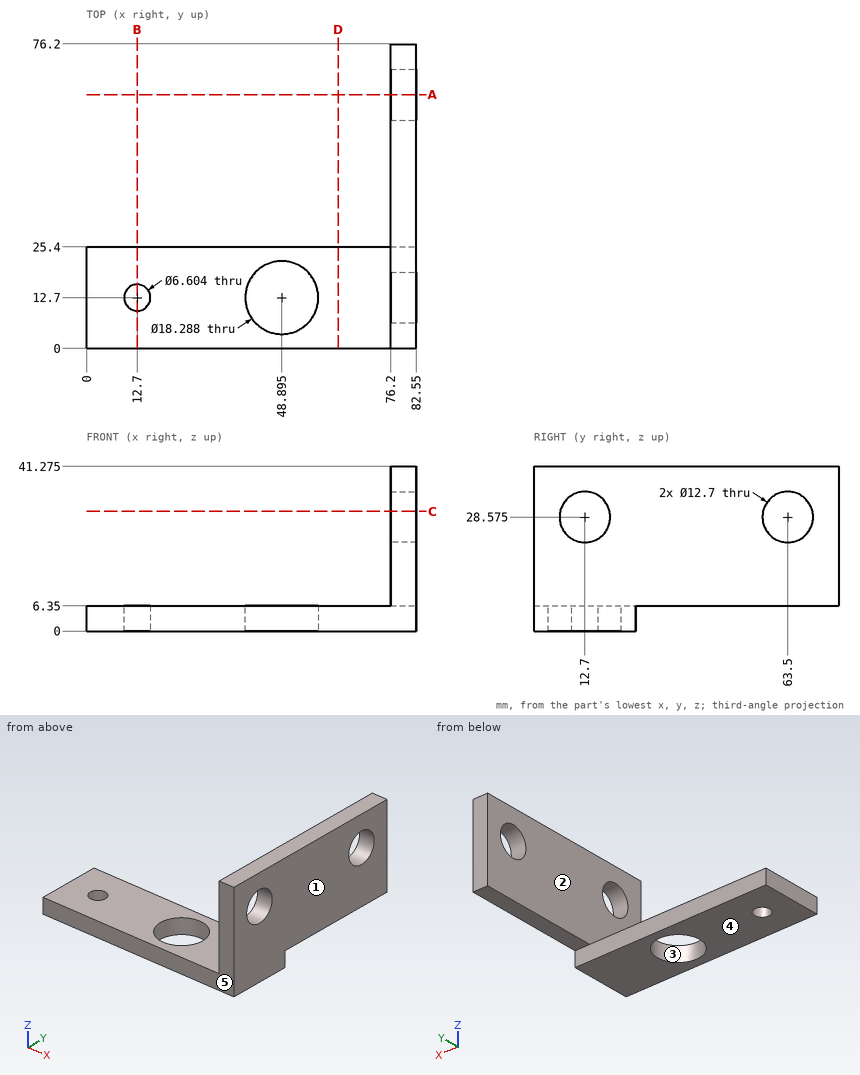
The figure shows three views and two pictorial views of one solid part (mm, origin at its lowest corner). Answer the questions. A direction names the side the tool comes from. Coordinates: 2 decimals unless noted, no trailing zeros. Write each loop counter-clockwise with the first axis right and the second up, starting at its lowest first coordinate (ties: lowest second). Pieces come first, ordered by that corner, then holes. Notation, with made-up numbers: M 20.25,-39.75 L 78.25,-39.75 A14 cw 78.25,-26.75 Z; hole C 68.25,-38.5 d8. An arc over 180 degrees is marked long. Answer as CSV lines item,"result". Start each with the question number.
Item 1: Section C-C on z = 30 is taken. Write down the section's boundary in (x, y).
Item 2: Consider L1, parallel to X at y = 71.5, z = 27; L2, parallel to Z at x = 79, y = 63 (3 decimals); L3, parallel to Z at x = 42.5, y = 24. Determine where each line is inside the solid, lowest interval first.
Item 3: Determine the mould class of the marked faces 3, 4 and 5 for opening direction Y: released by +Y, released by -Y, zero draft, split by the parting line, or undercut.
Item 4: Flat-ended cylindrical pins translate along their axes: P1, Ø8, axis at y = 40.5, z = 36, coming from the -X side; P2, Ø1.5, axis at x = 23, y = 20.5, coming from the +Z side; P3, Ø5, axis at x = 78.5, y = 54, coming from the -Z side; P4, Ø4, axis at x = 28, y = 26.5, coming from the -Z side. Find the tip coordinate at first contact, or state that the pin passes through.
Item 5: Section B-B on x = 12.7 is taken. Write down the section's boundary in (y, z), and give its area (3 significant figures).
Item 6: Section A-A on y = 63.5 is taken. Write down the section's boundary in (x, z) (3 decimals).
Item 7: Section D-D on x = 63 is taken. Write down the section's boundary in (y, z), and give its area (3 significant figures).
Item 8: A tool of negligible diameter and unlimited length cuts with its end or side. For the marked faces 1 and 2, from which of +Z, -Z, +X, -X, +Y, -Y can it reach the whole face along a straight path? Write none if from no direction.
Checks:
1,outline,"M 76.2,0 L 82.55,0 L 82.55,6.51 L 76.2,6.51 Z; M 76.2,18.89 L 82.55,18.89 L 82.55,57.31 L 76.2,57.31 Z; M 76.2,69.69 L 82.55,69.69 L 82.55,76.2 L 76.2,76.2 Z"
2,L1,"x = 76.2 to 82.55"
2,L2,"z = 6.35 to 22.245, 34.905 to 41.275"
2,L3,"z = 0 to 6.35"
3,face 3,"undercut"
3,face 4,"zero draft"
3,face 5,"released by -Y"
4,P1,"stops at x = 76.2"
4,P2,"stops at z = 6.35"
4,P3,"stops at z = 6.35"
4,P4,"stops at z = 0"
5,outline,"M 0,0 L 9.4,0 L 9.4,6.35 L 0,6.35 Z; M 16,0 L 25.4,0 L 25.4,6.35 L 16,6.35 Z"
5,area,"119 mm²"
6,outline,"M 76.2,6.35 L 82.55,6.35 L 82.55,22.225 L 76.2,22.225 Z; M 76.2,34.925 L 82.55,34.925 L 82.55,41.275 L 76.2,41.275 Z"
7,outline,"M 0,0 L 25.4,0 L 25.4,6.35 L 0,6.35 Z"
7,area,"161 mm²"
8,face 1,"+Z, -Z, +X, +Y, -Y"
8,face 2,"+Z, -X, +Y, -Y"
